For this review, take the finished solid that the model builds, in its own axes (mm). A direction names the side the tool comes from. Coordinates: 2 decimals unless noted, no trailing zeros. Order: outer loops, then holes, each group sorted by start corner. A loop starts at its lowest first (then second) coordinate and runs counter-clockwise, first axis right, second up. Notation, with made-up numbers: M 83.5,14 L 118.5,14 A8 cw 118.5,27 Z; hole C -33.5,49.25 d3. An arc over 180 degrees is marked long. Use CSV: the item, a comma, the result in double quotes.
```python
from build123d import *

# Parameters (mm, degrees)
BOSS_EXTRUDE2_DEPTH = 20
SKETCH4_R           = 5
BOSS_EXTRUDE3_DEPTH = 6
SKETCH5_R           = 5
CUT_EXTRUDE1_DEPTH  = 6


with BuildPart() as part:
    # Sketch3 → Boss-Extrude2 (new body)
    with BuildSketch(Plane(origin=(0, 0, 0), x_dir=(0, 0, -1), z_dir=(1, 0, 0))):
        with BuildLine():
            Line((100, -15), (-100, -15))
            ThreePointArc((-100, -15), (-115, 0), (-100, 15))
            Line((-100, 15), (100.0000001, 15))
            ThreePointArc((100.0000001, 15), (115.00000005, -5e-08), (100, -15))
        make_face()
    extrude(amount=BOSS_EXTRUDE2_DEPTH)

    # Sketch4 → Boss-Extrude3 (add)
    with BuildSketch(Plane(origin=(20, 0, 0), x_dir=(0, 0, -1), z_dir=(1, 0, 0))):
        with Locations((100.00000005, 0)):
            Circle(SKETCH4_R)
    boss_extrude3 = extrude(amount=BOSS_EXTRUDE3_DEPTH)

    # Sketch5 → Cut-Extrude1 (cut)
    with BuildSketch(Plane(origin=(20, 0, 0), x_dir=(0, 0, -1), z_dir=(1, 0, 0))):
        with Locations((-100, 0)):
            Circle(SKETCH5_R)
    cut_extrude1 = extrude(amount=-CUT_EXTRUDE1_DEPTH, mode=Mode.SUBTRACT)

    # Mirror1: Boss-Extrude3, Cut-Extrude1 across plane
    add(boss_extrude3.mirror(Plane(origin=(10, 0, 0), x_dir=(0, 0, 1), z_dir=(1, 0, 0))))
    add(cut_extrude1.mirror(Plane(origin=(10, 0, 0), x_dir=(0, 0, 1), z_dir=(1, 0, 0))), mode=Mode.SUBTRACT)


solid = part.part
```
Item 1: Clearance check with flat-ended pins moving along their axes: pin 1 Ø5 at (x, y) = (19, 3) entering from +Z; pin 2 Ø8 at (y, z) = (0, 100) entering from +X; pin 3 Ø5 at (y, z) = (-1.5, 99.5) entering from -X. State where each tip first meets the part, or that it passes through.
Solutions:
pin 1,"z = 114.99"
pin 2,"x = 14"
pin 3,"x = 6"
Item 2: To check wall thickness, follow line 1 along Y through (x, z) = (4, 100); line 2 along X through (y, z) = (8.5, -8); line 3 along Y through (x, z) = (18, -101). State the ranges of each line that lie inside material, in increasing order. Write a range as [from, to].
Solutions:
line 1,"[-15, -5], [5, 15]"
line 2,"[0, 20]"
line 3,"[-14.97, 14.97]"
Item 3: Add section A-A on y = 0. State the section outline as (x, z) points.
Solutions:
outline,"M -6,-105 L 0,-105 L 0,-115 L 20,-115 L 20,-105 L 26,-105 L 26,-95 L 20,-95 L 20,95 L 14,95 L 14,105 L 20,105 L 20,115 L 0,115 L 0,105 L 6,105 L 6,95 L 0,95 L 0,-95 L -6,-95 Z"
Item 4: For faces 1 (the face through (14, 0, 100)), 2 (the face through (2.958, -1.915, 95.381)), 3 (the face through (10, -15, -1)), list the 3-axis set-ups (+Z, -Z, +X, -X, +Y, -Y) from which the entire face can be reached by the end or side of a thin tool; tool diameter is ignored.
Solutions:
face 1,"+X"
face 2,"-X"
face 3,"+Z, -Z, +X, -X, -Y"
Item 5: Add section C-C on z = -85. State the section outline as (x, y) points, and give its area (3 significant figures).
Solutions:
outline,"M 0,-15 L 20,-15 L 20,15 L 0,15 Z"
area,"600 mm^2"
Item 6: Add section B-B on x = 8. State the section outline as (y, z) points.
Solutions:
outline,"M -15,-100 A15 ccw 15,-100 L 15,100 A15 ccw -15,100 Z"
Item 7: Draft analysis for pull direction Z (two halves, no side actions). For faces 4 (the face through (17.042, -1.915, 95.381)), 5 (the face through (-2.958, -1.915, -104.619)), 6 (the face through (0, 0, -2)), state which applies: released by +Z, released by -Z, zero draft, split by the parting line, or undercut.
Solutions:
face 4,"undercut"
face 5,"split by the parting line"
face 6,"zero draft"
